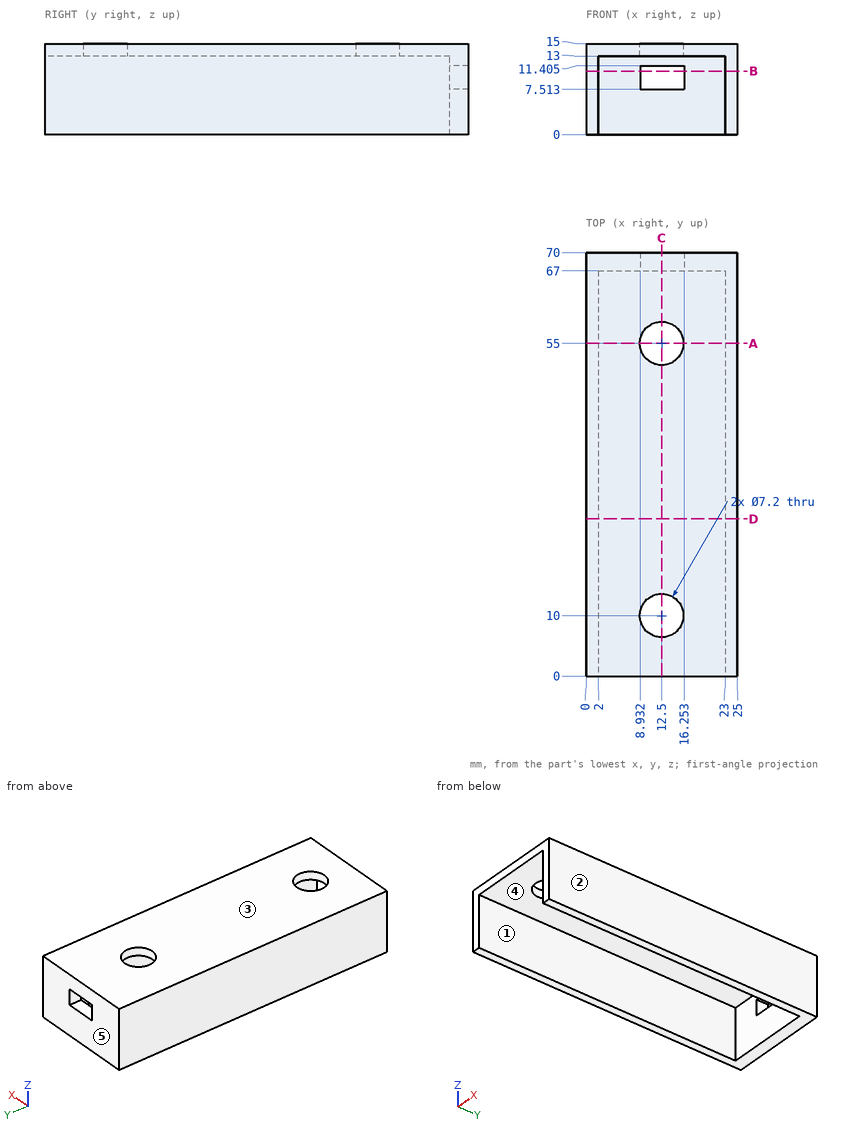
Here's the drawing with two shaded views (mm, measured from the low corner). I have some questions. A direction names the side the tool comes from. Round coordinates to 2 decimals unless told otherwise and drop trailing zeros. Write each loop counter-clockwise with the first axis right and the second up, starting at its lowest first coordinate (ties: lowest second). Pieces come first, ordered by that corner, then holes. Notation, with made-up numbers: M -32.75,-7 L -10.75,-7 A19 ccw -10.75,4 Z; hole C 67,7 d8. An arc over 180 degrees is marked long. Answer in a Markdown table with one row per item. Add a question column.
Q1. On a 3-axis mill with a long thin cutter (end or side, diameter ignored), from which of +Z, -Z, +X, -X, +Y, -Y can I reach the whole of each face in a straight line? I mean the marked faces 4 and 5. Say none if no direction works.
Q2. If I drill on line 1 (Y direction, x = 12.5, z = 14.2); line 2 (X direction, y = 29.5, z = 12.75); line 3 (Z direction, x = 20.5, y = 56), over which ranges is the centre line in solid material (lowest first)? Write a range as from..to.
Q3. If we mould it in two halves opening along X, with no side actions, what happens to the marked faces 1, 2 and 3? For each: +X half, -X half, draft (parallel to the pull), parting line (faces both ways), or undercut.
Q4. Imagine slicing it at A-A (y = 55). Please give me the cut outline in (x, z).
Q5. Will these pins go through, and if not, where does the flat tip stop? pin 1 Ø8 at (x, y) = (7.5, 21.5) entering from -Z; pin 2 Ø5 at (x, z) = (11, 13.5) entering from -Y; pin 3 Ø1.5 at (x, z) = (10.5, 7.5) entering from -Y.
Q6. Imagine slicing it at B-B (z = 10.5). Please give me the cut outline in (x, y).
Q7. Imagine slicing it at D-D (y = 26). Please give me the cut outline in (x, z).
Q8. Imagine slicing it at C-C (x = 12.5). Please give me the cut outline in (y, z) (1 decimal).
Values:
| question | item | result |
|---|---|---|
| 1 | face 4 | -Z, -Y |
| 1 | face 5 | +Z, -Z, +X, -X, +Y |
| 2 | line 1 | 0..6.4, 13.6..51.4, 58.6..70 |
| 2 | line 2 | 0..2, 23..25 |
| 2 | line 3 | 13..15 |
| 3 | face 1 | undercut |
| 3 | face 2 | +X half |
| 3 | face 3 | draft |
| 4 | outline | M 0,0 L 2,0 L 2,13 L 8.9,13 L 8.9,15 L 0,15 Z; M 16.1,13 L 23,13 L 23,0 L 25,0 L 25,15 L 16.1,15 Z |
| 5 | pin 1 | z = 13 |
| 5 | pin 2 | y = 0 |
| 5 | pin 3 | y = 67 |
| 6 | outline | M 0,0 L 2,0 L 2,67 L 8.93,67 L 8.93,70 L 0,70 Z; M 16.25,67 L 23,67 L 23,0 L 25,0 L 25,70 L 16.25,70 Z |
| 7 | outline | M 0,0 L 2,0 L 2,13 L 23,13 L 23,0 L 25,0 L 25,15 L 0,15 Z |
| 8 | outline | M 0,13 L 6.4,13 L 6.4,15 L 0,15 Z; M 13.6,13 L 51.4,13 L 51.4,15 L 13.6,15 Z; M 58.6,13 L 67,13 L 67,11.4 L 70,11.4 L 70,15 L 58.6,15 Z; M 67,0 L 70,0 L 70,7.5 L 67,7.5 Z |
